```python
from build123d import *

# Parameters (mm, degrees)
SKETCH_1_R      = 5
EXTRUDE_1_DEPTH = 65
EXTRUDE_START   = -10
SKETCH_1_3_R    = 8
SKETCH_1_3_R_2  = 5
EXTRUDE_2_DEPTH = 10
CHAMFER_1_SIZE  = 1


with BuildPart() as part:
    # Sketch 1 → Extrude 1 (new body)
    with BuildSketch(Plane.XY):
        Circle(SKETCH_1_R)
    extrude(amount=EXTRUDE_1_DEPTH)

    # Sketch 1_3 → Extrude 2 (add)
    # profile 1 of 2: a face of its own
    with BuildSketch(Plane.XY.offset(EXTRUDE_START)):
        Circle(SKETCH_1_3_R)
        Circle(SKETCH_1_3_R_2, mode=Mode.SUBTRACT)
    # profile 2 of 2: a face of its own
    with BuildSketch(Plane.XY.offset(EXTRUDE_START)):
        Circle(SKETCH_1_3_R_2)
    extrude(amount=EXTRUDE_2_DEPTH)

    # Chamfer 1
    chamfer_1_edges = [part.edges().sort_by_distance(p)[0] for p in [
        (-8, 0, -10),
    ]]
    chamfer(chamfer_1_edges, length=CHAMFER_1_SIZE)


solid = part.part
```
Input: part model. Units: mm. Frame: model coordinates. A direction names the side the tool comes from. Give positions to 0.01 mm unless a question says otherwise; leave off trailing zeros. Order: outer loops, then holes, each group sorted by start corner. A loop starts at its lowest first (then second) coordinate and runs counter-clockwise, first axis right, second up. Notation, with made-up numbers: M 54,-5 L 59,-5 A18 cw 59,19 Z; hole C -3.5,64 d11. An arc over 180 degrees is marked long. Return JSON: item names as keys, results as strings.
Item 1: Ray query, probe 1 along Z at (x, y) = (-5.5, 2); probe 2 along Y at (x, z) = (-0.25, -1); probe 3 along X at (y, z) = (-3.5, 61). Return the intervals inside material, ascending.
Solutions:
{"probe 1": "-10 to 0", "probe 2": "-8 to 8", "probe 3": "-3.57 to 3.57"}
Item 2: First-contact query: P1, Ø6, axis at y = 4.5, z = 46.5, coming from the +X side; P2, Ø5, axis at x = 5, z = 11, coming from the +Y side; P3, Ø3, axis at y = -3.5, z = 32.5, coming from the +X side. Flat tips, straight axial feed; report the tip coordinate or a pass-through.
Solutions:
{"P1": "x = 4.77", "P2": "y = 4.33", "P3": "x = 4.58"}
Item 3: Cut plane C-C (z = 59). Return loops of the section in (x, y), then the cut area to 3 significant figures.
Solutions:
{"outline": "C 0,0 d10", "area": "78.5 mm^2"}
Item 4: Cut plane A-A (y = 0). Return loops of the section in (x, z).
Solutions:
{"outline": "M -8,-9 L -7,-10 L 7,-10 L 8,-9 L 8,0 L 5,0 L 5,65 L -5,65 L -5,0 L -8,0 Z"}
Item 5: Access query for faces 1 (the cylindrical face through (-1.08, -4.88, 32.04)), 2 (the flat face through (0, 0, 65)). Directions: +Z, -Z, +X, -X, +Y, -Y. A direction counts if a zero-diameter tool reaches every point of the face in a straight line with its end or side. Return the directions, or none.
Solutions:
{"face 1": "+Z", "face 2": "+Z, +X, -X, +Y, -Y"}
